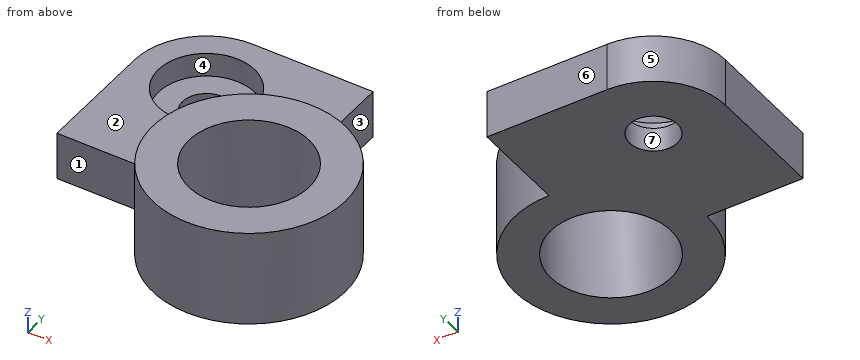
Autodesk Fusion 360 part; units mm, degrees
sketch "스케치1" plane through (0, 0, 0) normal (0, 0, 1) x (1, 0, 0)
  line L0 (0, 0) -> (40, 0)
  line L1 (40, 0) -> (40, 40)
  line L2 (40, 40) -> (15, 40)
  line L3 (0, 25) -> (0, 0)
  circle A0 centre (40, 0) radius 20
  circle A1 centre (40, 0) radius 12.5
  arc A2 (15, 40) -> (0, 25) centre (15, 25) ccw
  circle A3 centre (15, 25) radius 10
  circle A4 centre (15, 25) radius 5
  point P0 (0, 40)
  dimension "d1" = 40
  dimension "d2" = 40
  dimension "d3" = 40
  dimension "d4" = 25
  dimension "d5" = 15
  dimension "d6" = 20
  dimension "d7" = 10
extrude "돌출4" add sketch "스케치1" along normal blind 20 contours L0 L1 A0 A1 | L0 L1 A0 A1
extrude "돌출5" add sketch "스케치1" along normal blind 10 contours L0 L1 L2 L3 A0 A2
extrude "돌출6" add sketch "스케치1" along normal blind 5 contours A3
For this review, take the finished solid that the model builds, in its own axes (mm). Face numbers are marked on the shaded views. A direction names the side the tool comes from. Coordinates: 2 decimals unless noted, no trailing zeros. Write each loop counter-clockwise with the first axis right and the second up, starting at its lowest first coordinate (ties: lowest second). Pieces come first, ordered by that corner, then holes. Notation, with made-up numbers: (-11.75, 63.25) - (30.25, 63.25) arc R18 ccw to (30.25, 79.25) - close; hole circle Ø11 at (19, -3.75). An arc over 180 degrees is marked (long way). Put each result on its own line as item: value.
1. For pin 1 (10 mm diameter, centred on x = 15, y = 23.5, fed in from +Z); pin 2 (20 mm diameter, centred on x = 14, y = 27.5, fed in from +Z); pin 3 (5 mm diameter, centred on x = 9.5, z = 3.5, fed in from -Y), all flat-tipped, find the tip position at first contact; note any pin that passes through.
Values found:
pin 1: z = 5
pin 2: z = 10
pin 3: y = 0
2. Machinability: for the marked faces 1, 2, 3 and 4, which of the approach directions +Z, -Z, +X, -X, +Y, -Y give a long, thin tool a straight path to every point of the face, cutting with its end or side? Answer none if there is none.
Values found:
face 1: +Z, -Z, -X, -Y
face 2: +Z, -X, +Y
face 3: +Z, -Z, +X, +Y
face 4: +Z
3. Mouldability with a two-part tool opening along X and no side actions: class the marked faces 5, 6 and 7 as released by +X, released by -X, zero draft, split by the parting line, or undercut.
Values found:
face 5: released by -X
face 6: zero draft
face 7: undercut
4. Add section B-B, the plane x = 11. Give the boundary of the cut face in (y, z).
Values found:
outline: (0, 0) - (22, 0) - (22, 5) - (15.83, 5) - (15.83, 10) - (0, 10) - close; (28, 0) - (39.46, 0) - (39.46, 10) - (34.17, 10) - (34.17, 5) - (28, 5) - close
5. Add section D-D, the plane y = 31.5. Give the boundary of the cut face in (x, z).
Values found:
outline: (1.48, 0) - (40, 0) - (40, 10) - (22.6, 10) - (22.6, 5) - (7.4, 5) - (7.4, 10) - (1.48, 10) - close
6. Wall thickness on probe 1 along Y at (x, z) = (15, 1.1); probe 2 along Y at (x, z) = (40, 10.75); probe 3 along Z at (x, y) = (19, 9): over which ranges is each line inside the solid? List them lowest first.
Values found:
probe 1: 0 to 20, 30 to 40
probe 2: -20 to -12.5, 12.5 to 20
probe 3: 0 to 10
7. Add section A-A, the plane z = 3.5. Give the boundary of the cut face in (x, y).
Values found:
outline: (0, 0) - (20, 0) arc R20 ccw (long way) to (40, 20) - (40, 40) - (15, 40) arc R15 ccw to (0, 25) - close; hole circle Ø10 at (15, 25); hole circle Ø25 at (40, 0)
8. Add section C-C, the plane x = 24. Give the boundary of the cut face in (y, z), then the cut area to 3 significant figures.
Values found:
outline: (-12, 0) - (40, 0) - (40, 10) - (29.36, 10) - (29.36, 5) - (20.64, 5) - (20.64, 10) - (12, 10) - (12, 20) - (-12, 20) - close
area: 716 mm²
